Here's how the part is built. I have some questions about the finished solid (model axes, mm). A direction names the side the tool comes from. Coordinates: 2 decimals unless noted, no trailing zeros. Write each loop counter-clockwise with the first axis right and the second up, starting at its lowest first coordinate (ties: lowest second). Pieces come first, ordered by that corner, then holes. Notation, with made-up numbers: (83, 14) -> (112, 14) arc R13 ccw to (112, 39) -> close; hole circle Ø10 at (-10, 72). An arc over 180 degrees is marked (long way). Use a Markdown table: item, result. Add a question column.
Item 1: Will these pins go through, and if not, where does the flat tip stop? pin 1 Ø2 at (x, z) = (2, 5) entering from -Y; pin 2 Ø3.5 at (y, z) = (14.5, -1) entering from -X; pin 3 Ø6 at (x, z) = (-15, 0) entering from +Y; pin 4 Ø2 at (x, z) = (15.5, 0.5) entering from +Y.
Item 2: On a 3-axis mill with a long thin cutter (end or side, diameter ignored), from which of +Z, -Z, +X, -X, +Y, -Y can I reach the whole of each face in a straight line? I mean faces 4 (the flat face through (13, 10, 2)), 5 (the cylindrical face through (-0.225, 10.248, 0.098)). Say none if no direction works.
Item 3: If we mould it in two halves opening along Z, with no side actions, what happens to faces 1 (the flat face through (0, 12, 7)), 2 (the cylindrical face through (-12.854, 4.93, 0.676)), 3 (the flat face through (13, 0, 2))? For each: pulls with the +Z half, pulls with the -Z half, needs draft (parallel to the pull), parting line crosses it, or undercut.
Item 4: If I drill on line 1 along Z through (x, y) = (-15, 4); line 2 along X through (y, z) = (1.25, -1); line 3 along X through (y, z) = (2, 1.5), over which ranges is the centre line in solid material (lowest first)? Write a range as from..to.
Item 5: Imagine slicing it at B-B, the plane z = 0. Count the separate pieces of the cut face and the enclosed holes in it, and give its area (3 significant figures).
Item 6: Imagine slicing it at A-A, the plane y = 1.5. Write out the boundary of the cut face in (x, z).
```python
from build123d import *

# Parameters (mm, degrees)
BOSS_EXTRUDE1_DEPTH    = 7
FILLET1_R              = 2
SPLIT1_SURFACE_1_BACK  = 47.861
SPLIT1_SURFACE_1_DEPTH = 95.722
SPLIT1_SURFACE_2_BACK  = 47.861
SPLIT1_SURFACE_2_DEPTH = 95.722
CUT_EXTRUDE2_DEPTH     = 14
CUT_EXTRUDE8_DEPTH     = 32.559467847
SKETCH10_R             = 2.25
CUT_EXTRUDE6_DEPTH     = 35
CUT_EXTRUDE7_DEPTH     = 10
BOSS_EXTRUDE2_DEPTH    = 14


with BuildPart() as part:
    # Sketch1 → Boss-Extrude1 (new, symmetric)
    with BuildSketch(Plane.XY):
        with BuildLine():
            Line((10.25, 0), (20, 0))
            Line((20, 0), (20, 20))
            Line((20, 20), (-20, 20))
            Line((-20, 20), (-20, 0))
            Line((-20, 0), (-10.25, 0))
            ThreePointArc((-10.25, 0), (0, 10.25), (10.25, 0))
        make_face()
    extrude(amount=BOSS_EXTRUDE1_DEPTH, both=True)

    # Fillet1
    fillet1_edges = [part.edges().sort_by_distance(p)[0] for p in [
        (20, 0, 0),
        (-20, 0, 0),
    ]]
    fillet(fillet1_edges, radius=FILLET1_R)


with BuildPart() as body_2:
    # Split1: the piece behind the surface
    add(part.part)
    # Split1 surface: a surface, the sketch's curves swept straight by 95.722 mm
    with BuildLine(Plane.XY.offset(7).offset(-SPLIT1_SURFACE_1_BACK), mode=Mode.PRIVATE) as split1_surface_1_path:
        Line((0, 20), (0, 0))
    split1_surface_1 = Shell.extrude(split1_surface_1_path.wire(), (0 * SPLIT1_SURFACE_1_DEPTH, 0 * SPLIT1_SURFACE_1_DEPTH, 1 * SPLIT1_SURFACE_1_DEPTH))
    split(bisect_by=split1_surface_1, keep=Keep.BOTTOM)

    # Sketch6 → Cut-Extrude2 (cut)
    with BuildSketch(Plane.XY.offset(7)):
        with BuildLine():
            Line((-20, 20), (-20, 4.378237371))
            add(Edge.make_bspline(
                [(0, 20), (-18.821096643, 20), (-20, 4.378237371)],
                knots=[0, 0, 0, 0.882109664, 0.882109664, 0.882109664], degree=2))
            Line((0, 20), (-20, 20))
        make_face()
    extrude(amount=-CUT_EXTRUDE2_DEPTH, mode=Mode.SUBTRACT)


with BuildPart() as part_1:
    add(part.part)

    # Split1: split by a surface, the side it looks to stays
    # Split1 surface: a surface, the sketch's curves swept straight by 95.722 mm
    with BuildLine(Plane.XY.offset(7).offset(-SPLIT1_SURFACE_2_BACK), mode=Mode.PRIVATE) as split1_surface_2_path:
        Line((0, 20), (0, 0))
    split1_surface_2 = Shell.extrude(split1_surface_2_path.wire(), (0 * SPLIT1_SURFACE_2_DEPTH, 0 * SPLIT1_SURFACE_2_DEPTH, 1 * SPLIT1_SURFACE_2_DEPTH))
    split(bisect_by=split1_surface_2, keep=Keep.TOP)

    # Sketch6<3> → Cut-Extrude8 (cut, through all)
    with BuildSketch(Plane.XY.offset(7)):
        with BuildLine():
            Line((20, 20), (0, 20))
            add(Edge.make_bspline(
                [(0, 20), (18.821096643, 20), (20, 4.378237371)],
                knots=[0, 0, 0, 0.882109664, 0.882109664, 0.882109664], degree=2))
            Line((20, 4.378237371), (20, 20))
        make_face()
    extrude(amount=-CUT_EXTRUDE8_DEPTH, mode=Mode.SUBTRACT)


with BuildPart() as cut_extrude6_tool:
    # Sketch10 → Cut-Extrude6 (new body)
    with BuildSketch(Plane.XZ):
        with Locations((15, 0)):
            Circle(SKETCH10_R)
        with Locations((-15, 0)):
            Circle(SKETCH10_R)
    extrude(amount=-CUT_EXTRUDE6_DEPTH)


with BuildPart() as part_2:
    add(part_1.part)

    # Cut-Extrude6: cut by cut_extrude6_tool
    add(cut_extrude6_tool.part, mode=Mode.SUBTRACT)


with BuildPart() as body_2_1:
    add(body_2.part)

    # Cut-Extrude6: cut by cut_extrude6_tool
    add(cut_extrude6_tool.part, mode=Mode.SUBTRACT)


with BuildPart() as cut_extrude7_tool:
    # Sketch11 → Cut-Extrude7 (new body)
    with BuildSketch(Plane(origin=(0, 20, 0), x_dir=(1, 0, 0), z_dir=(0, 1, 0))):
        Polygon((-11.25, -2.165063509), (-11.25, 2.165063509), (-15, 4.330127019), (-18.75, 2.165063509), (-18.75, -2.165063509), (-15, -4.330127019), align=None)
        Polygon((15, -4.330127019), (11.25, -2.165063509), (11.25, 2.165063509), (15, 4.330127019), (18.75, 2.165063509), (18.75, -2.165063509), align=None)
    extrude(amount=-CUT_EXTRUDE7_DEPTH)


with BuildPart() as part_3:
    add(part_2.part)

    # Cut-Extrude7: cut by cut_extrude7_tool
    add(cut_extrude7_tool.part, mode=Mode.SUBTRACT)


with BuildPart() as body_2_2:
    add(body_2_1.part)

    # Cut-Extrude7: cut by cut_extrude7_tool
    add(cut_extrude7_tool.part, mode=Mode.SUBTRACT)

    # Combine1: union part
    add(part_3.part)

    # Sketch12 → Boss-Extrude2 (add)
    with BuildSketch(Plane.XY.offset(7)):
        with BuildLine():
            Line((-18, 0), (-20, 0))
            Line((-20, 0), (-20, 2))
            ThreePointArc((-20, 2), (-19.414213562, 0.585786438), (-18, 0))
        make_face()
        with BuildLine():
            Line((18, 0), (20, 0))
            Line((20, 0), (20, 2))
            ThreePointArc((20, 2), (19.414213562, 0.585786438), (18, 0))
        make_face()
    extrude(amount=-BOSS_EXTRUDE2_DEPTH)


solid = body_2_2.part
```
Ans:
| question | item | result |
|---|---|---|
| 1 | pin 1 | stops at y = 9.8 |
| 1 | pin 2 | stops at x = -12.26 |
| 1 | pin 3 | stops at y = 10 |
| 1 | pin 4 | passes through |
| 2 | face 4 | +Y |
| 2 | face 5 | +Z, -Z, -Y |
| 3 | face 1 | pulls with the +Z half |
| 3 | face 2 | undercut |
| 3 | face 3 | needs draft |
| 4 | line 1 | z = -7..-2.25, 2.25..7 |
| 4 | line 2 | x = -20..-17.02, -12.98..-10.17, 10.17..12.98, 17.02..20 |
| 4 | line 3 | x = -20..-16.68, -13.32..-10.05, 10.05..13.32, 16.68..20 |
| 5 | separate pieces | 3 |
| 5 | enclosed holes | 0 |
| 5 | area | 351 mm^2 |
| 6 | outline | (-20, -7) -> (-10.14, -7) -> (-10.14, 7) -> (-20, 7) -> close; (10.14, -7) -> (20, -7) -> (20, 7) -> (10.14, 7) -> close; hole circle Ø4.5 at (-15, 0); hole circle Ø4.5 at (15, 0) |
